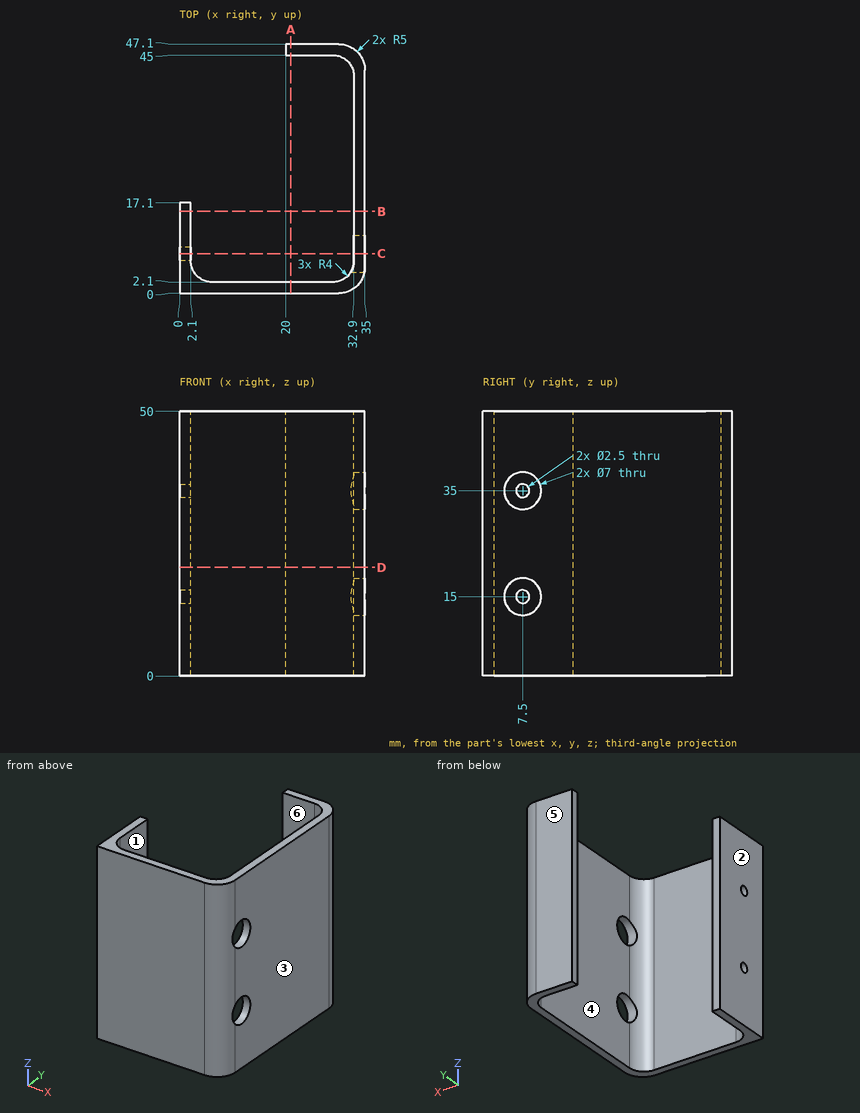
Could you check a few things on this drawing? It's one solid part, dimensions in mm from its lowest x, y, z. A direction names the side the tool comes from. Round coordinates to 2 decimals unless told otherwise and drop trailing zeros. Write each loop counter-clockwise with the first axis right and the second up, starting at its lowest first coordinate (ties: lowest second). Pieces come first, ordered by that corner, then holes. Notation, with made-up numbers: (26.5, 23) -> (67.5, 23) arc R14 cw to (67.5, 49) -> close; hole circle Ø11 at (32, 36.5). An arc over 180 degrees is marked (long way). Use one line per item in the form item = value. Start each with the question number.
Q1. I'm going to push flat-ended pins straight in: P1, Ø0.6, axis at x = 0.5, z = 24, coming from the +Y side; P2, Ø2, axis at x = 4.5, y = 9, coming from the +Z side; P3, Ø4, axis at y = 7.5, z = 15, coming from the +X side; P4, Ø4, axis at y = 26.5, z = 5, coming from the -X side. Where does each tip first touch, or does it pass through?
Q2. Imagine slicing it at A-A (x = 21). Please give me the cut outline in (y, z), then the cut area to 3 significant figures.
Q3. Imagine slicing it at C-C (y = 7.5). Please give me the cut outline in (x, z), then the cut area to 3 significant figures.
Q4. Imagine slicing it at D-D (z = 20.5). Please give me the cut outline in (x, y), then the cut area to 3 significant figures.
Q5. Which directions (+Z, -Z, +X, -X, +Y, -Y) give clear straight access to the entire face, cutting with the end or side of a thin tool? Please do the marked faces 4, 5 and 6.
Q6. Imagine slicing it at B-B (y = 15.5). Please give me the cut outline in (x, z).
Q7. If I drill on probe 1 along X at (y, z) = (14, 29.5); probe 2 along Y at (x, z) = (26.5, 39); probe 3 along X at (y, z) = (27, 39), over which ranges is the centre line in solid material (lowest first)? Write a range as [from, to].
Q8. We'd pull the mould along X, two halves only. Please class the marked faces 1, 2 and 3: +X half, -X half, draft (parallel to the pull), parting line (faces both ways), or undercut.
Worked out:
q1.P1 = 17.1
q1.P2 = through
q1.P3 = 2.15
q1.P4 = 32.9
q2.outline = (0, 0) -> (2.1, 0) -> (2.1, 50) -> (0, 50) -> close; (45, 0) -> (47.1, 0) -> (47.1, 50) -> (45, 50) -> close
q2.area = 210 mm^2
q3.outline = (0, 0) -> (2.1, 0) -> (2.1, 13.75) -> (0, 13.75) -> close; (0, 16.25) -> (2.1, 16.25) -> (2.1, 33.75) -> (0, 33.75) -> close; (0, 36.25) -> (2.1, 36.25) -> (2.1, 50) -> (0, 50) -> close; (32.9, 0) -> (35, 0) -> (35, 11.5) -> (32.9, 11.5) -> close; (32.9, 18.5) -> (35, 18.5) -> (35, 31.5) -> (32.9, 31.5) -> close; (32.9, 38.5) -> (35, 38.5) -> (35, 50) -> (32.9, 50) -> close
q3.area = 170 mm^2
q4.outline = (0, 0) -> (30, 0) arc R5 ccw to (35, 5) -> (35, 42.1) arc R5 ccw to (30, 47.1) -> (20, 47.1) -> (20, 45) -> (28.9, 45) arc R4 cw to (32.9, 41) -> (32.9, 6.1) arc R4 cw to (28.9, 2.1) -> (6.1, 2.1) arc R4 cw to (2.1, 6.1) -> (2.1, 17.1) -> (0, 17.1) -> close
q4.area = 226 mm^2
q5.face_4 = +Z, -Z
q5.face_5 = +Z, -Z, +X, -X, +Y
q5.face_6 = +Z, -Z, -X
q6.outline = (0, 0) -> (2.1, 0) -> (2.1, 50) -> (0, 50) -> close; (32.9, 0) -> (35, 0) -> (35, 50) -> (32.9, 50) -> close
q7.probe_1 = [0, 2.1], [32.9, 35]
q7.probe_2 = [0, 2.1], [45, 47.1]
q7.probe_3 = [32.9, 35]
q8.face_1 = undercut
q8.face_2 = -X half
q8.face_3 = +X half
